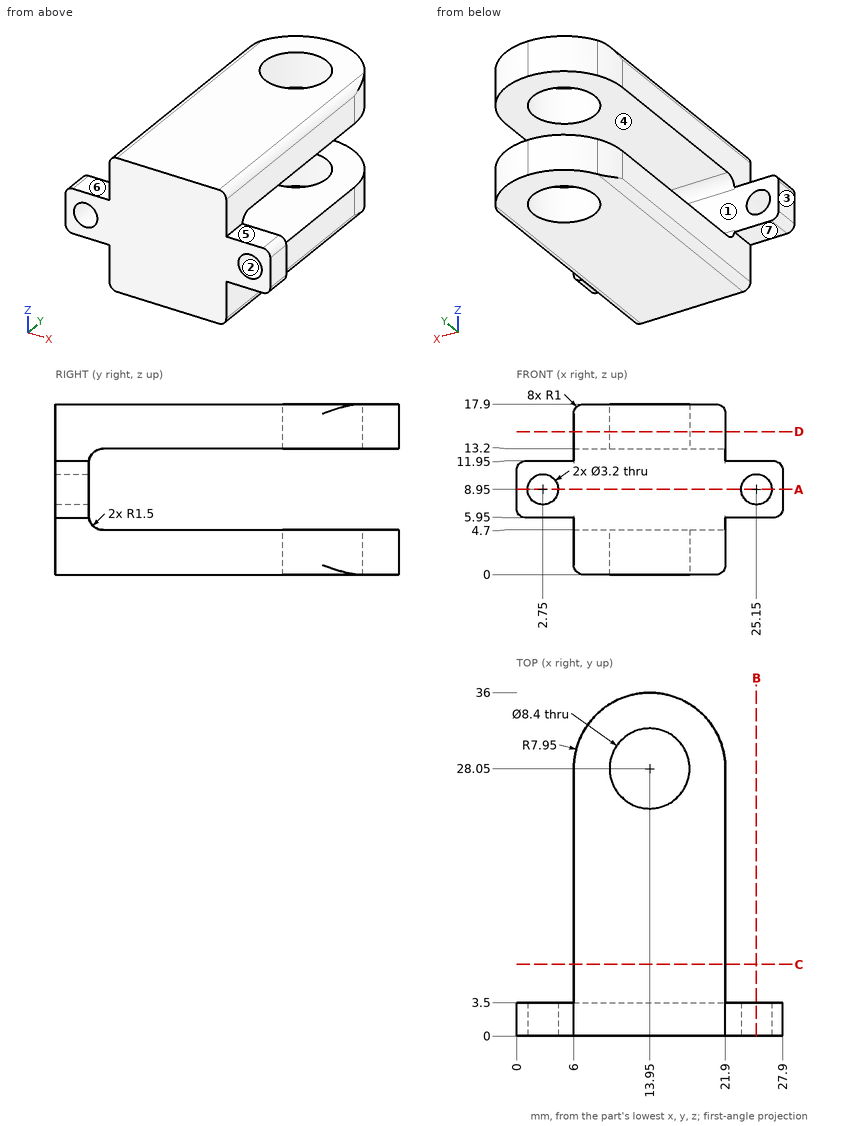
Here's the drawing with two shaded views (mm, measured from the low corner). I have some questions. A direction names the side the tool comes from. Round coordinates to 2 decimals unless told otherwise and drop trailing zeros. Write each loop counter-clockwise with the first axis right and the second up, starting at its lowest first coordinate (ties: lowest second). Pieces come first, ordered by that corner, then holes. Notation, with made-up numbers: M 54,88.25 L 103,88.25 A8 cw 103,92.25 Z; hole C -25,17 d9. An arc over 180 degrees is marked long. Answer in a Markdown table with one row per item. Add a question column.
Q1. On a 3-axis mill with a long thin cutter (end or side, diameter ignored), from which of +Z, -Z, +X, -X, +Y, -Y can I reach the whole of each face in a straight line? I mean the marked faces 4, 5, 6 and 7. Say none if no direction works.
Q2. Will these pins go through, and if not, where does the flat tip stop? pin 1 Ø5.5 at (y, z) = (18, 3) entering from +X; pin 2 Ø1.8 at (x, y) = (25, 2) entering from +Z; pin 3 Ø3 at (x, z) = (12.5, 8) entering from +Y; pin 4 Ø1 at (x, z) = (23, 15.5) entering from +Y.
Q3. If we mould it in two halves opening along X, with no side actions, what happens to the marked faces 1, 2 and 3? For each: +X half, -X half, draft (parallel to the pull), parting line (faces both ways), or undercut.
Q4. Imagine slicing it at B-B (x = 25.15). Please give me the cut outline in (y, z).
Q5. If I drill on line 1 (Y direction, x = 13.95, z = 1.4); line 2 (X direction, y = 1.7, z = 8.95); line 3 (Z direction, x = 18.25, y = 14.5), over which ranges is the centre line in solid material (lowest first)? Write a range as from..to.
Q6. Imagine slicing it at A-A (z = 8.95). Please give me the cut outline in (x, y).
Q7. Imagine slicing it at D-D (z = 15). Please give me the cut outline in (x, y).
Q8. Imagine slicing it at C-C (y = 7.5). Please give me the cut outline in (x, z).
Values:
| question | item | result |
|---|---|---|
| 1 | face 4 | +X, -X, +Y |
| 1 | face 5 | +Z, +X, +Y, -Y |
| 1 | face 6 | +Z, -X, +Y, -Y |
| 1 | face 7 | -Z, -X, +Y, -Y |
| 2 | pin 1 | x = 21.9 |
| 2 | pin 2 | z = 11.95 |
| 2 | pin 3 | y = 3.5 |
| 2 | pin 4 | through |
| 3 | face 1 | draft |
| 3 | face 2 | undercut |
| 3 | face 3 | -X half |
| 4 | outline | M 0,5.95 L 3.5,5.95 L 3.5,7.35 L 0,7.35 Z; M 0,10.55 L 3.5,10.55 L 3.5,11.95 L 0,11.95 Z |
| 5 | line 1 | 0..23.85, 32.25..36 |
| 5 | line 2 | 0..1.15, 4.35..23.55, 26.75..27.9 |
| 5 | line 3 | 0..4.7, 13.2..17.9 |
| 6 | outline | M 0,0 L 1.15,0 L 1.15,3.5 L 0,3.5 Z; M 4.35,0 L 23.55,0 L 23.55,3.5 L 4.35,3.5 Z; M 26.75,0 L 27.9,0 L 27.9,3.5 L 26.75,3.5 Z |
| 7 | outline | M 6,0 L 21.9,0 L 21.9,28.05 A7.95 ccw 6,28.05 Z; hole C 13.95,28.05 d8.4 |
| 8 | outline | M 6,1 A1 ccw 7,0 L 20.9,0 A1 ccw 21.9,1 L 21.9,4.7 L 6,4.7 Z; M 6,13.2 L 21.9,13.2 L 21.9,16.9 A1 ccw 20.9,17.9 L 7,17.9 A1 ccw 6,16.9 Z |
